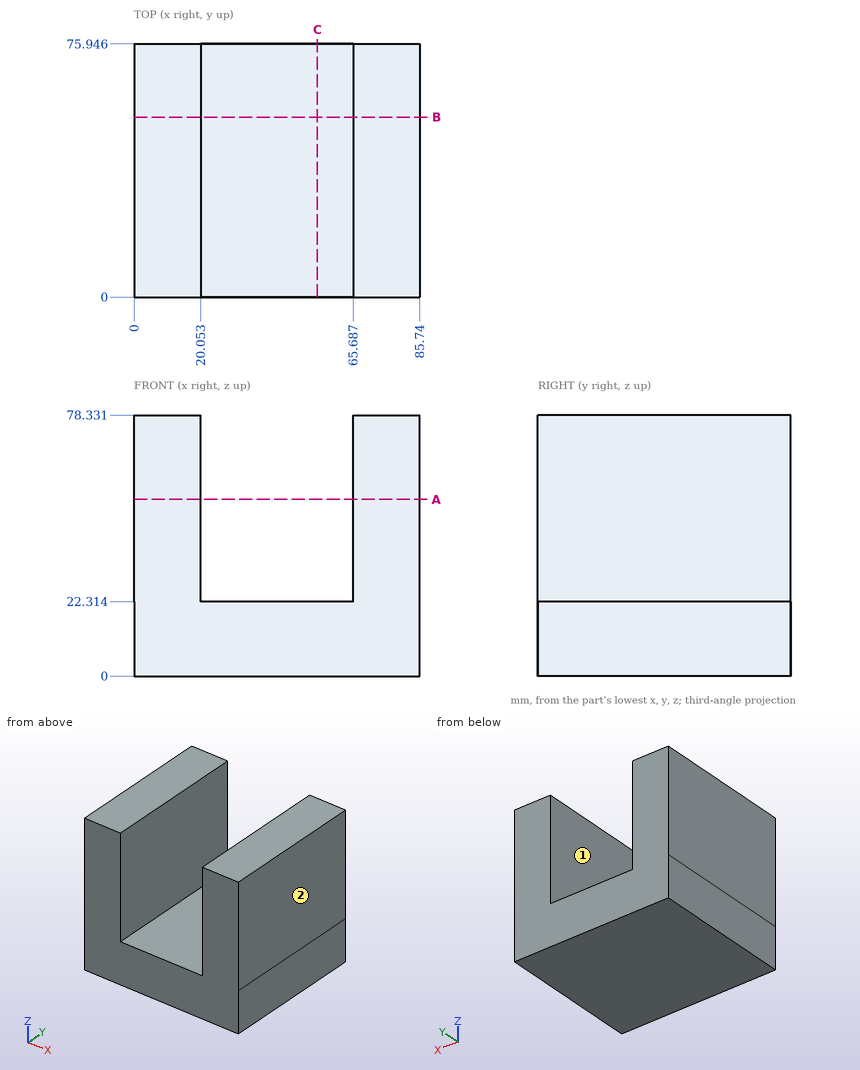
Here's the drawing with two shaded views (mm, measured from the low corner). I have some questions. A direction names the side the tool comes from. Coordinates: 2 decimals unless noted, no trailing zeros. Order: outer loops, then holes, each group sorted by start corner. A loop starts at its lowest first (then second) coordinate and runs counter-clockwise, first axis right, second up.
Item 1: Which directions (+Z, -Z, +X, -X, +Y, -Y) give clear straight access to the entire face, cutting with the end or side of a thin tool? Please do the marked faces 1 and 2.
Response values:
face 1: +Z, +Y, -Y
face 2: +Z, -Z, +X, +Y, -Y
Item 2: I need wall thicknesses on probe 1 along X at (y, z) = (64, 26.5); probe 2 along Z at (x, y) = (60, 16). Which ranges of each line are inside material? Lowest first, please.
Response values:
probe 1: x = 0 to 20.05, 65.69 to 85.74
probe 2: z = 0 to 22.31
Item 3: If we section it at A-A, the plane z = 53: List the corners of the cut face in (x, y) for me, then the cut area to 3 significant figures.
Response values:
outline: (0, 0) - (20.05, 0) - (20.05, 75.95) - (0, 75.95) - close; (65.69, 0) - (85.74, 0) - (85.74, 75.95) - (65.69, 75.95) - close
area: 3,050 mm2
Item 4: If we section it at C-C, the plane x = 55: List the corners of the cut face in (y, z) for me.
Response values:
outline: (0, 0) - (75.95, 0) - (75.95, 22.31) - (0, 22.31) - close
Item 5: If we section it at B-B, the plane y = 54: List the corners of the cut face in (x, z) for me.
Response values:
outline: (0, 0) - (85.74, 0) - (85.74, 78.33) - (65.69, 78.33) - (65.69, 22.31) - (20.05, 22.31) - (20.05, 78.33) - (0, 78.33) - close
Item 6: I'm going to push flat-ended pins straight in: pin 1 Ø1.5 at (x, z) = (63.5, 54) entering from +Y; pin 2 Ø13.5 at (x, y) = (35, 46.5) entering from +Z. Where does each tip first touch, or does it pass through?
Response values:
pin 1: passes through
pin 2: stops at z = 22.31
